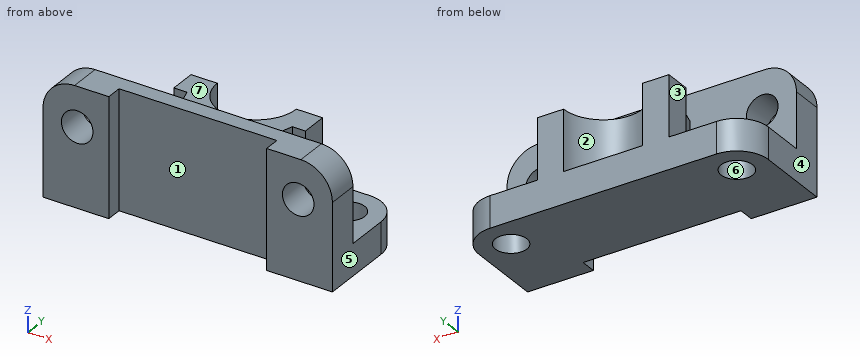
```python
from build123d import *

# Parameters (mm, degrees)
SKETCH1_W           = 110
SKETCH1_H           = 45
BOSS_EXTRUDE1_DEPTH = 12
FILLET1_R           = 12
SKETCH2_W           = 110
SKETCH2_H           = 28.361012769
BOSS_EXTRUDE2_DEPTH = 12
FILLET2_R           = 12
BOSS_EXTRUDE3_DEPTH = 23
SKETCH4_R           = 6
CUT_EXTRUDE1_DEPTH  = 66.845250742
SKETCH5_R           = 6
CUT_EXTRUDE2_DEPTH  = 76.782658648
SKETCH6_W           = 60
SKETCH6_H           = 6
CUT_EXTRUDE3_DEPTH  = 82.725218579


with BuildPart() as part:
    # Sketch1 → Boss-Extrude1 (new body)
    with BuildSketch(Plane(origin=(0, 0, 0), x_dir=(1, 0, 0), z_dir=(0, 1, 0))):
        Rectangle(SKETCH1_W, SKETCH1_H)
    extrude(amount=BOSS_EXTRUDE1_DEPTH)

    # Fillet1
    fillet1_edges = [part.edges().sort_by_distance(p)[0] for p in [
        (55, 6, 22.5),
        (-55, 6, 22.5),
    ]]
    fillet(fillet1_edges, radius=FILLET1_R)

    # Sketch2 → Boss-Extrude2 (add)
    with BuildSketch(Plane(origin=(0, 0, -22.5), x_dir=(-1, 0, 0), z_dir=(0, 0, -1))):
        with Locations((0, 26.180506385)):
            Rectangle(SKETCH2_W, SKETCH2_H)
    extrude(amount=-BOSS_EXTRUDE2_DEPTH)

    # Fillet2
    fillet2_edges = [part.edges().sort_by_distance(p)[0] for p in [
        (55, 40.361012769, -16.5),
        (-55, 40.361012769, -16.5),
    ]]
    fillet(fillet2_edges, radius=FILLET2_R)

    # Sketch3 → Boss-Extrude3 (add)
    with BuildSketch(Plane.XY.offset(-10.5)):
        with BuildLine():
            Line((15, 40.361012769), (25, 40.361012769))
            Line((25, 40.361012769), (25, 30.361012769))
            Line((25, 30.361012769), (20, 30.361012769))
            Line((20, 30.361012769), (11, 0))
            Line((11, 0), (-11, 0))
            Line((-11, 0), (-20, 30.361012769))
            Line((-20, 30.361012769), (-25, 30.361012769))
            Line((-25, 30.361012769), (-25, 40.361012769))
            Line((-25, 40.361012769), (-15, 40.361012769))
            ThreePointArc((-15, 40.361012769), (0, 25.361012769), (15, 40.361012769))
        make_face()
    extrude(amount=BOSS_EXTRUDE3_DEPTH)

    # Sketch4 → Cut-Extrude1 (cut, through all)
    with BuildSketch(Plane(origin=(0, 12, 0), x_dir=(1, 0, 0), z_dir=(0, 1, 0))):
        with Locations(Location((-42, -7.5, 0), (0, 0, 270))):
            Circle(SKETCH4_R)
        with Locations(Location((42, -7.5, 0), (0, 0, 270))):
            Circle(SKETCH4_R)
    extrude(amount=-CUT_EXTRUDE1_DEPTH, mode=Mode.SUBTRACT)

    # Sketch5 → Cut-Extrude2 (cut, through all)
    with BuildSketch(Plane.XY.offset(-10.5)):
        with Locations((-43, 28.361012769)):
            Circle(SKETCH5_R)
        with Locations(Location((42.820569124, 28.361012769, 0), (0, 0, 180))):
            Circle(SKETCH5_R)
    extrude(amount=-CUT_EXTRUDE2_DEPTH, mode=Mode.SUBTRACT)

    # Sketch6 → Cut-Extrude3 (cut, through all)
    with BuildSketch(Plane.XY.offset(22.5)):
        with Locations((0, 3)):
            Rectangle(SKETCH6_W, SKETCH6_H)
    extrude(amount=-CUT_EXTRUDE3_DEPTH, mode=Mode.SUBTRACT)


solid = part.part
```
Build history of the part. All positions in model axes, mm. Face numbers are marked on the shaded views. A direction names the side the tool comes from. Give positions to 0.01 mm unless a question says otherwise; leave off trailing zeros. Loops run counter-clockwise (first coordinate to the right, second up) from the corner with the lowest first, then second, coordinate; pieces in that order, holes last.
Item 1: Flat gauge pins, fed straight in: pin 1 (8.5 mm diameter, centred on x = -10, y = 32.5, fed in from +Z); pin 2 (11 mm diameter, centred on y = 38, z = -2.5, fed in from +X); pin 3 (10 mm diameter, centred on y = 17.5, z = 8.5, fed in from -X). Where does each tip first touch, or does it go through?
Answers follow:
pin 1: stops at z = 12.5
pin 2: stops at x = 25
pin 3: stops at x = -17.67
Item 2: Slice it at A-A, the plane z = 7.5. List the corners of the cut face in (x, y), and give its area (3 significant figures).
Answers follow:
outline: (-55, 0) - (-48, 0) - (-48, 12) - (-55, 12) - close; (-36, 0) - (-30, 0) - (-30, 6) - (30, 6) - (30, 0) - (36, 0) - (36, 12) - (14.56, 12) - (20, 30.36) - (25, 30.36) - (25, 40.36) - (15, 40.36) arc R15 cw to (-15, 40.36) - (-25, 40.36) - (-25, 30.36) - (-20, 30.36) - (-14.56, 12) - (-36, 12) - close; (48, 0) - (55, 0) - (55, 12) - (48, 12) - close
area: 1,450 mm2
Item 3: Pull direction X, two halves, no side cores. Call the marked faces 4, 5, 6 and 7: released by +X, released by -X, zero draft, split by the parting line, or undercut.
Answers follow:
face 4: released by -X
face 5: released by +X
face 6: undercut
face 7: zero draft
Item 4: Slice it at D-D, the plane z = -14.5. List the corners of the cut face in (x, y).
Answers follow:
outline: (-55, 0) - (-30, 0) - (-30, 6) - (30, 6) - (30, 0) - (55, 0) - (55, 28.36) arc R12 ccw to (43, 40.36) - (-43, 40.36) arc R12 ccw to (-55, 28.36) - close; hole circle Ø12 at (-43, 28.36); hole circle Ø12 at (42.82, 28.36)
Item 5: Drill centre lines: line 1 (X direction, y = 4, z = 7); line 2 (X direction, y = 6.5, z = 7.5); line 3 (X direction, y = 26, z = -13.5). Where is each one in solid material? Low to high.
Answers follow:
line 1: x = -55 to -47.98, -36.02 to -30, 30 to 36.02, 47.98 to 55
line 2: x = -55 to -48, -36 to 36, 48 to 55
line 3: x = -55 to -48.52, -37.48 to 37.3, 48.34 to 55
Item 6: Slice it at B-B, the plane y = 8.5. List the corners of the cut face in (x, z).
Answers follow:
outline: (-55, -22.5) - (55, -22.5) - (55, 10.5) arc R12 ccw to (43, 22.5) - (-43, 22.5) arc R12 ccw to (-55, 10.5) - close; hole circle Ø12 at (-42, 7.5); hole circle Ø12 at (42, 7.5)
Item 7: Which spindle directions (+Z, -Z, +X, -X, +Y, -Y) get a long thin tool onto all of the face, cutting with end or side? Do the marked faces 1, 2 and 3. Say none if no direction does.
Answers follow:
face 1: +Z, -Z, -Y
face 2: +Z, +Y
face 3: +Z, -X, +Y
Item 8: Slice it at C-C, the plane y = 32.5. List the corners of the cut face in (x, z).
Answers follow:
outline: (-54.26, -22.5) - (-47.34, -22.5) - (-47.34, -10.5) - (-54.26, -10.5) - close; (-38.66, -22.5) - (38.48, -22.5) - (38.48, -10.5) - (25, -10.5) - (25, 12.5) - (12.78, 12.5) - (12.78, -10.5) - (-12.78, -10.5) - (-12.78, 12.5) - (-25, 12.5) - (-25, -10.5) - (-38.66, -10.5) - close; (47.16, -22.5) - (54.26, -22.5) - (54.26, -10.5) - (47.16, -10.5) - close
